from build123d import *

# Parameters (mm, degrees)
SKETCH_1_W             = 36.5
SKETCH_1_H             = 60
SM_BASE_FLANGE_1_DEPTH = 2
SM_START               = -30
SM_EDGE_FLANGE_1_DEPTH = 60
CUT_EXTRUDE_1_DEPTH    = 10
SKETCH_17_R            = 1.5
CUT_EXTRUDE_2_DEPTH    = 54.518688325


# Read off the part's stored shape, not the designer's step: 邊線-凸緣1
# Sheet-metal steps are written as plain solids
with BuildPart() as part:
    # Sketch 1 → 基材-凸緣1 (new body)
    with BuildSketch(Plane.XY):
        Rectangle(SKETCH_1_W, SKETCH_1_H)
    extrude(amount=-SM_BASE_FLANGE_1_DEPTH)

    # 邊線-凸緣1 outline → 邊線-凸緣1 (add)
    with BuildSketch(Plane(origin=(0, 0, 0), x_dir=(1, 0, 0), z_dir=(0, 1, 0)).offset(SM_START)):
        with BuildLine():
            ThreePointArc((20.25, 0), (19.664213562, 1.414213562), (18.25, 2))
            Line((18.25, 2), (18.25, -18))
            Line((18.25, -18), (20.25, -18))
            Line((20.25, -18), (20.25, 0))
        make_face()
        with BuildLine():
            Line((-20.25, 0), (-20.25, -18))
            Line((-20.25, -18), (-18.25, -18))
            Line((-18.25, -18), (-18.25, 2))
            ThreePointArc((-18.25, 2), (-19.664213562, 1.414213562), (-20.25, 0))
        make_face()
    extrude(amount=SM_EDGE_FLANGE_1_DEPTH)

    # 草圖14 → 除料-伸長1 (cut)
    with BuildSketch(Plane(origin=(0, 0, -2), x_dir=(-1, 0, 0), z_dir=(0, 0, -1))):
        with BuildLine():
            Line((-8.173166384, 25), (8.173166384, 25))
            ThreePointArc((8.173166384, 25), (9.91716134, 23.979020733), (9.880573604, 21.958481596))
            Line((9.880573604, 21.958481596), (1.70740722, 8.559848179))
            ThreePointArc((1.70740722, 8.559848179), (0, 7.601366583), (-1.70740722, 8.559848179))
            Line((-1.70740722, 8.559848179), (-9.880573604, 21.958481596))
            ThreePointArc((-9.880573604, 21.958481596), (-9.91716134, 23.979020733), (-8.173166384, 25))
        make_face()
        with BuildLine():
            Line((-15.25, 12.119944893), (-15.25, -12.119944893))
            ThreePointArc((-15.25, -12.119944893), (-13.79091846, -14.045407751), (-11.54259278, -13.161463297))
            Line((-11.54259278, -13.161463297), (-4.149426396, -1.041518404))
            ThreePointArc((-4.149426396, -1.041518404), (-3.856833616, 0), (-4.149426396, 1.041518404))
            Line((-4.149426396, 1.041518404), (-11.54259278, 13.161463297))
            ThreePointArc((-11.54259278, 13.161463297), (-13.79091846, 14.045407751), (-15.25, 12.119944893))
        make_face()
        with BuildLine():
            Line((-8.173166384, -25), (8.173166384, -25))
            ThreePointArc((8.173166384, -25), (9.91716134, -23.979020733), (9.880573604, -21.958481596))
            Line((9.880573604, -21.958481596), (1.70740722, -8.559848179))
            ThreePointArc((1.70740722, -8.559848179), (0, -7.601366583), (-1.70740722, -8.559848179))
            Line((-1.70740722, -8.559848179), (-9.880573604, -21.958481596))
            ThreePointArc((-9.880573604, -21.958481596), (-9.91716134, -23.979020733), (-8.173166384, -25))
        make_face()
        with BuildLine():
            Line((13.25, 8.841256368), (13.25, -8.841256368))
            ThreePointArc((13.25, -8.841256368), (11.79091846, -10.766719227), (9.54259278, -9.882774772))
            Line((9.54259278, -9.882774772), (4.149426396, -1.041518404))
            ThreePointArc((4.149426396, -1.041518404), (3.856833616, 0), (4.149426396, 1.041518404))
            Line((4.149426396, 1.041518404), (9.54259278, 9.882774772))
            ThreePointArc((9.54259278, 9.882774772), (11.79091846, 10.766719227), (13.25, 8.841256368))
        make_face()
    extrude(amount=-CUT_EXTRUDE_1_DEPTH, mode=Mode.SUBTRACT)

    # 草圖17 → 除料-伸長2 (cut, through all)
    with BuildSketch(Plane(origin=(20.25, 0, 0), x_dir=(0, 0, -1), z_dir=(1, 0, 0))):
        with Locations((-3, 25)):
            Circle(SKETCH_17_R)
        with Locations((-3, -25)):
            Circle(SKETCH_17_R)
        with Locations((-3, 0)):
            Circle(SKETCH_17_R)
    extrude(amount=-CUT_EXTRUDE_2_DEPTH, mode=Mode.SUBTRACT)


solid = part.part
Model file for the job. Use its own axes, mm. A direction names the side the tool comes from. Give positions to 0.01 mm unless a question says otherwise; leave off trailing zeros. Write each loop counter-clockwise with the first axis right and the second up, starting at its lowest first coordinate (ties: lowest second). Pieces come first, ordered by that corner, then holes. Notation, with made-up numbers: M 61.25,-38 L 79.25,-38 A27 ccw 79.25,-1 Z; hole C 73.25,-34 d11. An arc over 180 degrees is marked long. One line per item, written item: value. Start each with the question number.
Q1. Two-plate mould, pull along Z, no slides. Class faces 3 (the cylindrical face through (-19.65, -0.42, -1.43)), 4 (the cylindrical face through (-19.236, 26.487, 3.195)), 5 (the cylindrical face through (13.756, 14.055, -1.014)): +Z half, -Z half, draft (parallel to the pull), parting line (faces both ways), or undercut.
Q2. 3-axis set-ups, long thin cutter, end or side, ignore diameter. For faces 1 (the flat face through (20.25, 0, 9)), 2 (the flat face through (0, 25, -1)): which of +Z, -Z, +X, -X, +Y, -Y reach the whole face in a straight line?
Q3. Saw through at D-D, the plane z = 10. Write the cut outline in (x, y), plus the area to 3 significant figures.
Q4. Saw through at A-A, the plane z = 3. State how many separate pieces and enclosed holes the cut face has, plus the area to 3 significant figures.
Q5. Saw through at C-C, the plane x = 14.5. Write the cut outline in (y, z), plus the area to 3 significant figures.
Q6. Saw through at B-B, the plane y = 0. Write the cut outline in (x, z), plus the area to 3 significant figures.
Q7. Drop flat-ended pins along their axis: pin 1 Ø10 at (x, y) = (9.5, 20.5) entering from +Z; pin 2 Ø1.8 at (y, z) = (25, 3) entering from -X; pin 3 Ø0.6 at (y, z) = (-1, -0.5) entering from -X. Give the stop position or say it passes through.
Q8. Probe probe 1 along Y at (x, z) = (-18.9, 3); probe 2 along X at (y, z) = (-7, 8.25); probe 3 along X at (y, z) = (11, -0.75). List the from-to ranges inside material, lowest first. Write a range as [from, to].
Output values:
1. face 3: -Z half
1. face 4: undercut
1. face 5: draft
2. face 1: +Z, -Z, +X, +Y, -Y
2. face 2: +Z, -Z
3. outline: M -20.25,-30 L -18.25,-30 L -18.25,30 L -20.25,30 Z; M 18.25,-30 L 20.25,-30 L 20.25,30 L 18.25,30 Z
3. area: 240 mm²
4. separate pieces: 8
4. enclosed holes: 0
4. area: 204 mm²
5. outline: M -30,-2 L -13.68,-2 L -13.68,0 L -30,0 Z; M 13.68,-2 L 30,-2 L 30,0 L 13.68,0 Z
5. area: 65.3 mm²
6. outline: M -20.25,0 A2 ccw -18.25,-2 L -13.25,-2 L -13.25,0 L -18.25,0 L -18.25,1.5 L -20.25,1.5 Z; M -20.25,4.5 L -18.25,4.5 L -18.25,18 L -20.25,18 Z; M -3.86,-2 L 3.86,-2 L 3.86,0 L -3.86,0 Z; M 15.25,-2 L 18.25,-2 A2 ccw 20.25,0 L 20.25,1.5 L 18.25,1.5 L 18.25,0 L 15.25,0 Z; M 18.25,4.5 L 20.25,4.5 L 20.25,18 L 18.25,18 Z
6. area: 97.7 mm²
7. pin 1: stops at z = 0
7. pin 2: passes through
7. pin 3: stops at x = -20.24
8. probe 1: y = [-30, -26.5], [-23.5, -1.5], [1.5, 23.5], [26.5, 30]
8. probe 2: x = [-20.25, -18.25], [18.25, 20.25]
8. probe 3: x = [-20.1, -3.2], [3.2, 10.22], [15.25, 20.1]
